```python
from build123d import *

# Parameters (mm, degrees)
ESQUISSE1_W                  = 20
ESQUISSE1_H                  = 12
BOSS_EXTRU_1_DEPTH           = 15
ESQUISSE1_4_R                = 4
ENL_V_MAT_EXTRU_1_DEPTH      = 12
CONG_2_R                     = 4
ENL_V_MAT_EXTRU_2_DEPTH      = 54.749418763
ENL_V_MAT_EXTRU_2_DEPTH_BACK = 10
ESQUISSE2_R                  = 2.75
ESQUISSE4_R                  = 3.5
ENL_V_MAT_EXTRU_3_DEPTH      = 1
ESQUISSE5_R                  = 3.5
ENL_V_MAT_EXTRU_4_DEPTH      = 1


with BuildPart() as part:
    # Esquisse1 → Boss.-Extru.1 (new body)
    with BuildSketch(Plane(origin=(0, 0, 0), x_dir=(1, 0, 0), z_dir=(0, 1, 0))):
        Polygon((-38, 12), (-42, 8), (-42, -8), (-38, -12), (38, -12), (42, -8), (42, 8), (38, 12), (22, 12), (14, 18), (-14, 18), (-22, 12), align=None)
        with Locations((0, 3)):
            Rectangle(ESQUISSE1_W, ESQUISSE1_H, mode=Mode.SUBTRACT)
    extrude(amount=BOSS_EXTRU_1_DEPTH)

    # Congé1
    # a fillet whose section is not a circle: 4 mm, written as the material it adds along each edge
    with BuildSketch(Plane(origin=(22, 0, -12), x_dir=(1, 0, 0), z_dir=(0, 1, 0)), Plane(origin=(-22, 0, -12), x_dir=(0.7999999999999996, 0, -0.6000000000000003), z_dir=(0, 1, 0))) as cong_1_piece_1:
        with BuildLine():
            add(Edge.make_bspline([(1.333333333, 0), (1.087283439, 0), (0.841233545, 0), (0.292751215, 0.037020099), (-0.211988912, 0.205266808), (-0.672986836, 0.504740127), (-0.869826751, 0.652370064), (-1.066666667, 0.8)], knots=[0, 0, 0, 0, 0, 0, 0.5, 0.5, 1, 1, 1, 1, 1, 1], degree=5))
            Line((-1.066666667, 0.8), (0, 0))
            Line((0, 0), (1.333333333, 0))
        make_face()
    extrude(amount=15)
    # a fillet whose section is not a circle: 4 mm, written as the material it takes off along each edge
    with BuildSketch(Plane(origin=(42, -4.142135624, 8), x_dir=(-0.707106781186547, 0, 0.7071067811865481), z_dir=(0, 1, 0)), Plane(origin=(38, -4.142135624, 12), x_dir=(-1, 0, 0), z_dir=(0, 1, 0)), Plane(origin=(42, -4.142135624, -8), x_dir=(0, 0, 1), z_dir=(0, 1, 0)), Plane(origin=(38, -4.142135624, -12), x_dir=(0.7071067811865481, 0, 0.707106781186547), z_dir=(0, 1, 0)), Plane(origin=(-42, -4.142135624, -8), x_dir=(0.7071067811865475, 0, -0.7071067811865475), z_dir=(0, 1, 0)), Plane(origin=(-42, -4.142135624, 8), x_dir=(0, 0, -1), z_dir=(0, 1, 0)), Plane(origin=(-38, -4.142135624, 12), x_dir=(-0.7071067811865465, 0, -0.7071067811865486), z_dir=(0, 1, 0))) as cong_1_2_piece_1:
        with BuildLine():
            add(Edge.make_bspline([(1.656854249, 0), (1.35356905, 0), (1.050283851, 0), (0.373674798, -0.056927592), (-0.223974097, -0.30448187), (-0.742662833, -0.742662833), (-0.957117854, -0.957117854), (-1.171572875, -1.171572875)], knots=[0, 0, 0, 0, 0, 0, 0.5, 0.5, 1, 1, 1, 1, 1, 1], degree=5))
            Line((-1.171572875, -1.171572875), (0, 0))
            Line((0, 0), (1.656854249, 0))
        make_face()
    extrude(amount=23.284271247, mode=Mode.SUBTRACT)
    with BuildSketch(Plane(origin=(14, -3.333333333, -18), x_dir=(0.7999999999999996, 0, 0.6000000000000003), z_dir=(0, 1, 0)), Plane(origin=(-14, -3.333333333, -18), x_dir=(1, 0, 0), z_dir=(0, 1, 0))) as cong_1_2_piece_2:
        with BuildLine():
            add(Edge.make_bspline([(1.333333333, 0), (1.087283439, 0), (0.841233545, 0), (0.292751215, -0.037020099), (-0.211988912, -0.205266808), (-0.672986836, -0.504740127), (-0.869826751, -0.652370064), (-1.066666667, -0.8)], knots=[0, 0, 0, 0, 0, 0, 0.5, 0.5, 1, 1, 1, 1, 1, 1], degree=5))
            Line((-1.066666667, -0.8), (0, 0))
            Line((0, 0), (1.333333333, 0))
        make_face()
    extrude(amount=21.666666667, mode=Mode.SUBTRACT)
    with BuildSketch(Plane(origin=(-38, -4.142135624, -12), x_dir=(-0.7071067811865465, 0, 0.7071067811865486), z_dir=(0, 1, 0))) as cong_1_2_piece_3:
        with BuildLine():
            add(Edge.make_bspline([(1.656854249, 0), (1.35356905, 0), (1.050283851, 0), (0.373674798, 0.056927592), (-0.223974097, 0.30448187), (-0.742662833, 0.742662833), (-0.957117854, 0.957117854), (-1.171572875, 1.171572875)], knots=[0, 0, 0, 0, 0, 0, 0.5, 0.5, 1, 1, 1, 1, 1, 1], degree=5))
            Line((-1.171572875, 1.171572875), (0, 0))
            Line((0, 0), (1.656854249, 0))
        make_face()
    extrude(amount=23.284271247, mode=Mode.SUBTRACT)

    # Esquisse1<4> → Enlèv. mat.-Extru.1 (cut)
    with BuildSketch(Plane(origin=(0, 0, 0), x_dir=(1, 0, 0), z_dir=(0, 1, 0))):
        with Locations(Location((-30, 0, 0), (0, 0, 270))):
            Circle(ESQUISSE1_4_R)
        with Locations(Location((30, 0, 0), (0, 0, 270))):
            Circle(ESQUISSE1_4_R)
    extrude(amount=ENL_V_MAT_EXTRU_1_DEPTH, mode=Mode.SUBTRACT)

    # Congé2
    cong_2_edges = [part.edges().sort_by_distance(p)[0] for p in [
        (-10, 7.5, -9),
        (-10, 7.5, 3),
        (10, 7.5, 3),
        (10, 7.5, -9),
    ]]
    fillet(cong_2_edges, radius=CONG_2_R)

    # Esquisse2 → Enlèv. mat.-Extru.2 (cut, two sides: drawn at the far end of the back side and taken through both)
    with BuildSketch(Plane.XY.offset(12).offset(-ENL_V_MAT_EXTRU_2_DEPTH_BACK)):
        with Locations(Location((-28.75, 7.5, 0), (0, 0, 180))):
            Circle(ESQUISSE2_R)
        with Locations(Location((28.75, 7.5, 0), (0, 0, 180))):
            Circle(ESQUISSE2_R)
    extrude(amount=ENL_V_MAT_EXTRU_2_DEPTH + ENL_V_MAT_EXTRU_2_DEPTH_BACK, mode=Mode.SUBTRACT)

    # Esquisse4 → Enlèv. mat.-Extru.3 (cut)
    with BuildSketch(Plane.XY.offset(12)):
        with Locations((28.75, 7.5)):
            Circle(ESQUISSE4_R)
    extrude(amount=-ENL_V_MAT_EXTRU_3_DEPTH, mode=Mode.SUBTRACT)

    # Esquisse5 → Enlèv. mat.-Extru.4 (cut)
    with BuildSketch(Plane.XY.offset(12)):
        with Locations((-28.75, 7.5)):
            Circle(ESQUISSE5_R)
    extrude(amount=-ENL_V_MAT_EXTRU_4_DEPTH, mode=Mode.SUBTRACT)


solid = part.part
```
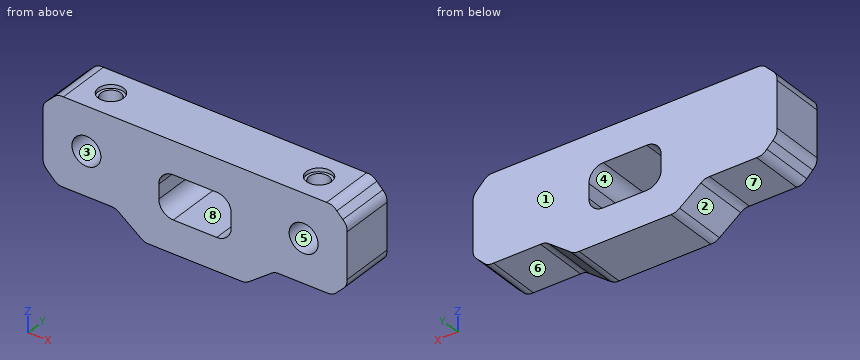
CAD build for the part. Positions are in the model's coordinates, mm. Face numbers are marked on the shaded views. A direction names the side the tool comes from. Round coordinates to 2 decimals unless told otherwise and drop trailing zeros. Write each loop counter-clockwise with the first axis right and the second up, starting at its lowest first coordinate (ties: lowest second). Pieces come first, ordered by that corner, then holes. Notation, with made-up numbers: (51.5, 66) - (58.5, 66) arc R10 cw to (58.5, 83) - close; hole circle Ø5 at (71, -31.75). An arc over 180 degrees is marked (long way). Return JSON: item names as keys, results as strings. Group by question number.
Item 1: Mould opens along Z. For the marked faces 1, 2, 3 and 4 say: +Z half, -Z half, draft (parallel to the pull), parting line (faces both ways), or undercut.
Item 2: 3-axis set-ups, long thin cutter, end or side, ignore diameter. For the marked faces 5, 6, 7 and 8: which of +Z, -Z, +X, -X, +Y, -Y reach the whole face in a straight line?
Item 3: Band-saw the part on C-C on x = 28.75. List the corners of the cut face in (y, z).
Item 4: Probe probe 1 along Y at (x, z) = (-28.75, 6.75); probe 2 along X at (y, z) = (4.5, 0); probe 3 along Z at (x, y) = (3, 14.75). List the from-to ranges inside material, lowest first.
Item 5: Flat gauge pins, fed straight in: pin 1 Ø6.5 at (x, y) = (32, 7.5) entering from -Z; pin 2 Ø5 at (x, z) = (30, 0) entering from -Y; pin 3 Ø6.5 at (x, z) = (31, -1) entering from -Y; pin 4 Ø6 at (x, y) = (-24.5, 7) entering from -Z. Where does each tip first touch, or does it go through?
Item 6: Band-saw the part on A-A on x = -1. List the corners of the cut face in (y, z).
Item 7: Band-saw the part on D-D on z = -15. List the corners of the cut face in (x, y), plus the area to 3 significant figures.
Item 8: Band-saw the part on B-B on z = 0. List the corners of the cut face in (x, y), plus the area to 3 significant figures.
Resolved:
{
 "1": {"face 1": "draft", "face 2": "-Z half", "face 3": "undercut", "face 4": "undercut"},
 "2": {"face 5": "-Y", "face 6": "-Z, +X, +Y, -Y", "face 7": "-Z, -X, +Y, -Y", "face 8": "+Y, -Y"},
 "3": {"outline": "(0, -12) - (15, -12) - (15, 12) - (11, 12) - (11, 11) - (10.25, 11) - (10.25, 3.8) - (12, 3.8) - (12, -3.8) - (0, -3.8) - close; (0, 3.8) - (4.75, 3.8) - (4.75, 11) - (4, 11) - (4, 12) - (0, 12) - close"},
 "4": {"probe 1": "y = 0 to 4.75, 10.25 to 15", "probe 2": "x = -42 to -34, -26 to -9.87, 9.87 to 26, 34 to 42", "probe 3": "z = -18 to -9, 3 to 12"},
 "5": {"pin 1": "stops at z = -12", "pin 2": "stops at y = 12", "pin 3": "stops at y = 0", "pin 4": "stops at z = -12.41"},
 "6": {"outline": "(0, -18) - (15, -18) - (15, -9) - (0, -9) - close; (0, 3) - (15, 3) - (15, 12) - (0, 12) - close"},
 "7": {"outline": "(-18, 0) - (18, 0) - (18, 15) - (-18, 15) - close", "area": "540 mm²"},
 "8": {"outline": "(-42, 0) - (-34, 0) - (-34, 12) - (-26, 12) - (-26, 0) - (-9.87, 0) - (-9.87, 15) - (-42, 15) - close; (9.87, 0) - (26, 0) - (26, 12) - (34, 12) - (34, 0) - (42, 0) - (42, 15) - (9.87, 15) - close", "area": "772 mm²"}
}
